CAD build for the part. Positions are in the model's coordinates, mm. A direction names the side the tool comes from. Round coordinates to 2 decimals unless told otherwise and drop trailing zeros. Order: outer loops, then holes, each group sorted by start corner. A loop starts at its lowest first (then second) coordinate and runs counter-clockwise, first axis right, second up. Notation, with made-up numbers: (30, 40) - (44, 40) arc R25 cw to (44, 66) - close; hole circle Ø11 at (-31.5, -23). An arc over 180 degrees is marked (long way). Write item = value, one per line.
from build123d import *

# Parameters (mm, degrees)
SKETCH1_W          = 55
SKETCH1_H          = 28
PCB_DEPTH          = 1.6
SKETCH2_W          = 55
SKETCH2_H          = 2.5
HEADER_A_DEPTH     = 8.5
SKETCH3_W          = 55
SKETCH3_H          = 2.5
HEADER_B_DEPTH     = 8.5
SKETCH4_W          = 18.5
SKETCH4_H          = 18
WROOM_MODULE_DEPTH = 3.2
SKETCH5_W          = 7.5
SKETCH5_H          = 8
USB_DEPTH          = 3


with BuildPart() as part:
    # Sketch1 → PCB (new body)
    with BuildSketch(Plane.XY):
        Rectangle(SKETCH1_W, SKETCH1_H)
    extrude(amount=PCB_DEPTH)

    # Sketch2 → Header_A (add)
    with BuildSketch(Plane.XY.offset(-8.5)):
        with Locations((0, -12.75)):
            Rectangle(SKETCH2_W, SKETCH2_H)
    extrude(amount=HEADER_A_DEPTH)

    # Sketch3 → Header_B (add)
    with BuildSketch(Plane.XY.offset(-8.5)):
        with Locations((0, 12.75)):
            Rectangle(SKETCH3_W, SKETCH3_H)
    extrude(amount=HEADER_B_DEPTH)

    # Sketch4 → WROOM_module (add)
    with BuildSketch(Plane.XY.offset(1.6)):
        with Locations((18.25, 0)):
            Rectangle(SKETCH4_W, SKETCH4_H)
    extrude(amount=WROOM_MODULE_DEPTH)

    # Sketch5 → USB (add)
    with BuildSketch(Plane.XY.offset(1.6)):
        with Locations((-25.75, 0)):
            Rectangle(SKETCH5_W, SKETCH5_H)
    extrude(amount=USB_DEPTH)


solid = part.part
(1) Band-saw the part on D-D on z = 3. List the corners of the cut face in (x, y).
Solved:
outline = (-29.5, -4) - (-22, -4) - (-22, 4) - (-29.5, 4) - close; (9, -9) - (27.5, -9) - (27.5, 9) - (9, 9) - close
(2) Band-saw the part on C-C on x = -13. List the corners of the cut face in (y, z), plus the area to 3 significant figures.
Solved:
outline = (-14, -8.5) - (-11.5, -8.5) - (-11.5, 0) - (11.5, 0) - (11.5, -8.5) - (14, -8.5) - (14, 1.6) - (-14, 1.6) - close
area = 87.3 mm²
(3) Probe line 1 along Y through (x, z) = (-14, -0.5); line 2 along Z through (x, y) = (-24.5, 9.75); line 3 along X through (y, z) = (4, 0.25). List the from-to ranges inside material, lowest first.
Solved:
line_1 = -14 to -11.5, 11.5 to 14
line_2 = 0 to 1.6
line_3 = -27.5 to 27.5
(4) Band-saw the part on A-A on z = -6.75. List the corners of the cut face in (x, y).
Solved:
outline = (-27.5, -14) - (27.5, -14) - (27.5, -11.5) - (-27.5, -11.5) - close; (-27.5, 11.5) - (27.5, 11.5) - (27.5, 14) - (-27.5, 14) - close
(5) Drop flat-ended pins along their axis: pin 1 (1.5 mm diameter, centred on y = -9.5, z = 1, fed in from -X); pin 2 (2.5 mm diameter, centred on x = 15, z = 3.5, fed in from +Y); pin 3 (8.5 mm diameter, centred on x = 1.5, y = 1, fed in from +Z). Give the stop position or say it passes through.
Solved:
pin_1 = -27.5
pin_2 = 9
pin_3 = 1.6
(6) Pull direction Y, two halves, no side cores. Call faces 4 (the flat face through (18, 0, 4.8)), 5 (the flat face through (0, -11.5, -4)), 6 (the flat face through (0, -14, -4)): released by +Y, released by -Y, zero draft, split by the parting line, or undercut.
Solved:
face_4 = zero draft
face_5 = undercut
face_6 = released by -Y
(7) Band-saw the part on B-B on y = 1.5. List the corners of the cut face in (x, z).
Solved:
outline = (-29.5, 1.6) - (-27.5, 1.6) - (-27.5, 0) - (27.5, 0) - (27.5, 4.8) - (9, 4.8) - (9, 1.6) - (-22, 1.6) - (-22, 4.6) - (-29.5, 4.6) - close
(8) Tool access for faces 1 (the flat face through (9, 0, 3)), 2 (the flat face through (-26, 0, 4.6)), 3 (the flat face through (0, 0, 0)): list every direction of +Z, -Z, +X, -X, +Y, -Y with a clear straight run to the whole face (end or side of a thin tool).
Solved:
face_1 = +Z, +Y, -Y
face_2 = +Z, -X, +Y, -Y
face_3 = -Z, +X, -X
